```python
from build123d import *

# Parameters (mm, degrees)
SKETCH2_W           = 212
SKETCH2_H           = 130
BOSS_EXTRUDE1_DEPTH = 3
BOSS_EXTRUDE2_DEPTH = 4


with BuildPart() as part:
    # Sketch2 → Boss-Extrude1 (new body)
    with BuildSketch(Plane(origin=(0, 0, 0), x_dir=(1, 0, 0), z_dir=(0, 1, 0))):
        Rectangle(SKETCH2_W, SKETCH2_H)
    extrude(amount=BOSS_EXTRUDE1_DEPTH)

    # Sketch3 → Boss-Extrude2 (add)
    with BuildSketch(Plane(origin=(0, 3, 0), x_dir=(1, 0, 0), z_dir=(0, 1, 0))):
        Polygon((91, 53.5), (77, 53.5), (77, 49.5), (87, 49.5), (87, 39.5), (91, 39.5), align=None)
        Polygon((91, -39.5), (91, -53.5), (77, -53.5), (77, -49.5), (87, -49.5), (87, -39.5), align=None)
        Polygon((-43, -49.5), (-43, -39.5), (-47, -39.5), (-47, -53.5), (-33, -53.5), (-33, -49.5), align=None)
        Polygon((-43, 39.5), (-47, 39.5), (-47, 53.5), (-33, 53.5), (-33, 49.5), (-43, 49.5), align=None)
    extrude(amount=BOSS_EXTRUDE2_DEPTH)


solid = part.part
```
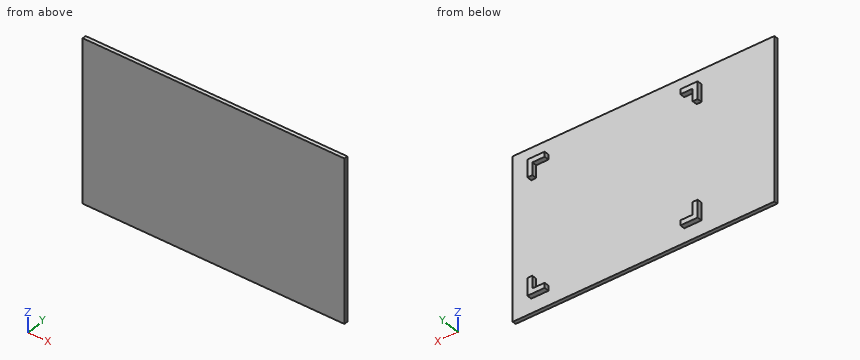
Design review of the part built by this model. Coordinates are the model's own, in mm. Coordinates: 2 decimals unless noted, no trailing zeros. Write each loop counter-clockwise with the first axis right and the second up, starting at its lowest first coordinate (ties: lowest second). Pieces come first, ordered by that corner, then holes.
1) Insertion check: pin 1 (1.2 mm diameter, centred on x = 87, y = 6, fed in from -Z); pin 2 (1.2 mm diameter, centred on x = -44, y = 5.5, fed in from +Z); pin 3 (1.2 mm diameter, centred on y = 5.5, z = 46.5, fed in from +X). Each pin has a flat end and moves straight along its axis. Give the tip position at first contact, or say it passes through.
2) Add section A-A (y = 4.75). Write out the cut boundary in (x, z), plus the area to 3 significant figures.
3) To check wall thickness, follow L1, parallel to X at y = 4.25, z = -43.5; L2, parallel to Y at x = -45.5, z = 55.5. State the ranges of each line that lie inside material, in increasing order.
4) Add section D-D (z = -29). Write out the cut boundary in (x, y).
5) Add section B-B (z = 47). Write out the cut boundary in (x, y), plus the area to 3 significant figures.
6) Add section C-C (x = 53.5). Write out the cut boundary in (y, z), plus the area to 3 significant figures.
Check result:
1. pin 1: stops at z = -53.5
1. pin 2: stops at z = 53.5
1. pin 3: stops at x = 91
2. outline: (-47, -53.5) - (-33, -53.5) - (-33, -49.5) - (-43, -49.5) - (-43, -39.5) - (-47, -39.5) - close; (-47, 39.5) - (-43, 39.5) - (-43, 49.5) - (-33, 49.5) - (-33, 53.5) - (-47, 53.5) - close; (77, -53.5) - (91, -53.5) - (91, -39.5) - (87, -39.5) - (87, -49.5) - (77, -49.5) - close; (77, 49.5) - (87, 49.5) - (87, 39.5) - (91, 39.5) - (91, 53.5) - (77, 53.5) - close
2. area: 384 mm2
3. L1: x = -47 to -43, 87 to 91
3. L2: y = 0 to 3
4. outline: (-106, 0) - (106, 0) - (106, 3) - (-106, 3) - close
5. outline: (-106, 0) - (106, 0) - (106, 3) - (91, 3) - (91, 7) - (87, 7) - (87, 3) - (-43, 3) - (-43, 7) - (-47, 7) - (-47, 3) - (-106, 3) - close
5. area: 668 mm2
6. outline: (0, -65) - (3, -65) - (3, 65) - (0, 65) - close
6. area: 390 mm2
